Read the model definition and answer for the solid it produces. Units are mm, in the model's axes. Face numbers are marked on the shaded views. A direction names the side the tool comes from. Coordinates: 2 decimals unless noted, no trailing zeros. Loops run counter-clockwise (first coordinate to the right, second up) from the corner with the lowest first, then second, coordinate; pieces in that order, holes last. Notation, with made-up numbers: M 48,33 L 102,33 A30 cw 102,70 Z; hole C 31,87.25 d4. An arc over 180 degrees is marked long. Use one line per item in the form item = value. Start each with the question number.
1. Flat-ended cylindrical pins translate along their axes: pin 1 (5 mm diameter, centred on x = 48, y = -45, fed in from -Z); pin 2 (2 mm diameter, centred on x = -17, y = -13, fed in from -Z); pin 3 (11 mm diameter, centred on x = -3, z = 63, fed in from +Y). Find the tip coordinate at first contact, or state that the pin passes through.
2. The part is cut by section C-C (y = -4.5). Give the vertices of the cut face in (x, z).
3. The part is cut by section B-B (x = 0). Give the vertices of the cut face in (y, z), plus the area to 3 significant figures.
4. A tool of negligible diameter and unlimited length cuts with its end or side. For the marked faces 5 and 6, from which of +Z, -Z, +X, -X, +Y, -Y can it reach the whole face along a straight path? Write none if from no direction.
5. For a pull along X with two mould halves and no side action, classify the marked faces 1, 2, 3 and 4 as released by +X, released by -X, zero draft, split by the parting line, or undercut.
6. The part is cut by section A-A (z = 0). Give the vertices of the cut face in (x, y).
7. The part is cut by section D-D (y = -39). Give the vertices of the cut face in (x, z), plus the area to 3 significant figures.
8. Find the intervals of material crossed by probe 1 along Z at (x, y) = (0, -26); probe 2 along X at (y, z) = (-39.5, -2), in increasing order. Write a range as [from, to].
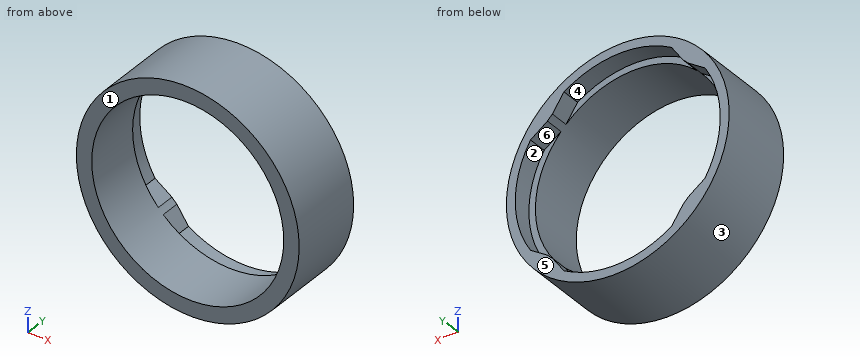
from build123d import *

# Parameters (mm, degrees)
SKETCH1_R           = 76.2
SKETCH1_R_2         = 65.659
BOSS_EXTRUDE1_DEPTH = 50.8
CUT_EXTRUDE1_DEPTH  = 12.7
CIRPATTERN1_COUNT   = 4


with BuildPart() as part:
    # Sketch1 → Boss-Extrude1 (new body)
    with BuildSketch(Plane(origin=(0, 0, 0), x_dir=(1, 0, 0), z_dir=(0, 1, 0))):
        Circle(SKETCH1_R)
        Circle(SKETCH1_R_2, mode=Mode.SUBTRACT)
    extrude(amount=-BOSS_EXTRUDE1_DEPTH)

    # Sketch2 → Cut-Extrude1 (cut)
    with BuildSketch(Plane(origin=(0, 0, 0), x_dir=(1, 0, 0), z_dir=(0, 1, 0))):
        with BuildLine():
            Line((-48.080896893, -44.713886377), (-59.672253185, -36.793926344))
            ThreePointArc((-59.672253185, -36.793926344), (-70.104, 0), (-59.672253185, 36.793926344))
            Line((-59.672253185, 36.793926344), (-48.080896893, 44.713886377))
            ThreePointArc((-48.080896893, 44.713886377), (-65.659, 0), (-48.080896893, -44.713886377))
        make_face()
    cut_extrude1 = extrude(amount=-CUT_EXTRUDE1_DEPTH, mode=Mode.SUBTRACT)

    # CirPattern1: Cut-Extrude1 ×4 about axis
    cirpattern1_axis = Axis((0, 0, 0), (0, 1, 0))
    for i in range(1, CIRPATTERN1_COUNT):
        add(cut_extrude1.rotate(cirpattern1_axis, i * 360 / CIRPATTERN1_COUNT), mode=Mode.SUBTRACT)


solid = part.part
Computed values:
q1.pin_1 = -61.12
q1.pin_2 = -74.5
q1.pin_3 = -12.7
q2.outline = C 0,0 d152.4; hole M -59.67,-36.79 L -48.08,-44.71 A65.66 ccw -44.71,-48.08 L -36.79,-59.67 A70.1 ccw 36.79,-59.67 L 44.71,-48.08 A65.66 ccw 48.08,-44.71 L 59.67,-36.79 A70.1 ccw 59.67,36.79 L 48.08,44.71 A65.66 ccw 44.71,48.08 L 36.79,59.67 A70.1 ccw -36.79,59.67 L -44.71,48.08 A65.66 ccw -48.08,44.71 L -59.67,36.79 A70.1 ccw Z
q3.outline = M -50.8,-76.2 L 0,-76.2 L 0,-70.1 L -12.7,-70.1 L -12.7,-65.66 L -50.8,-65.66 Z; M -50.8,65.66 L -12.7,65.66 L -12.7,70.1 L 0,70.1 L 0,76.2 L -50.8,76.2 Z
q3.area = 958 mm²
q4.face_5 = +Z, -Z, +X, -X, +Y
q4.face_6 = +Y
q5.face_1 = zero draft
q5.face_2 = undercut
q5.face_3 = split by the parting line
q5.face_4 = undercut
q6.outline = M -76.2,-50.8 L -65.66,-50.8 L -65.66,-12.7 L -70.1,-12.7 L -70.1,0 L -76.2,0 Z; M 65.66,-50.8 L 76.2,-50.8 L 76.2,0 L 70.1,0 L 70.1,-12.7 L 65.66,-12.7 Z
q7.outline = C 0,0 d152.4; hole C 0,0 d131.32
q7.area = 4,700 mm²
q8.probe_1 = [-76.2, -65.66], [65.66, 76.2]
q8.probe_2 = [-76.17, -65.63], [65.63, 76.17]
